```python
from build123d import *
from build123d.topology import SkipClean

# Parameters (mm, degrees)
SKETCH_1_R           = 15
SKETCH_1_R_2         = 4
SKETCH_1_R_3         = 1.6
EXTRUDE_1_DEPTH      = 4
EXTRUDE_START        = -4
EXTRUDE_3_DEPTH      = 4
EXTRUDE_4_DEPTH      = 8
EXTRUDE_4_DEPTH_BACK = 12
CUT_EXTRUDE_1_DEPTH  = 46


with BuildPart() as part:
    # 草图1 → 凸台-拉伸1 (new body)
    with BuildSketch(Plane.XY):
        Circle(SKETCH_1_R)
        Circle(SKETCH_1_R_2, mode=Mode.SUBTRACT)
        with Locations((0, 8)):
            Circle(SKETCH_1_R_3, mode=Mode.SUBTRACT)
        with Locations((6.92820323, 4)):
            Circle(SKETCH_1_R_3, mode=Mode.SUBTRACT)
        with Locations((6.92820323, -4)):
            Circle(SKETCH_1_R_3, mode=Mode.SUBTRACT)
        with Locations((0, -8)):
            Circle(SKETCH_1_R_3, mode=Mode.SUBTRACT)
        with Locations((-6.92820323, -4)):
            Circle(SKETCH_1_R_3, mode=Mode.SUBTRACT)
        with Locations((-6.92820323, 4)):
            Circle(SKETCH_1_R_3, mode=Mode.SUBTRACT)
    extrude(amount=EXTRUDE_1_DEPTH)

    # 草图2 → 凸台-拉伸3 (add)
    with BuildSketch(Plane.XY.offset(4).offset(EXTRUDE_START)):
        with BuildLine():
            Line((16.8, 85), (16.8, 54.159799849))
            ThreePointArc((16.8, 54.159799849), (15.83854762, 48.033324147), (13.046629547, 42.49587991))
            ThreePointArc((13.046629547, 42.49587991), (7.420814059, 25.504374344), (12.472191289, 8.333333333))
            ThreePointArc((12.472191289, 8.333333333), (-5.937882388, 13.774670695), (-14.621995932, -3.346226976))
            ThreePointArc((-14.621995932, -3.346226976), (-15.737901413, 44.738127218), (2.117573463, 89.398315084))
            ThreePointArc((2.117573463, 89.398315084), (11.095712057, 92.663530919), (16.8, 85))
        make_face()
    extrude(amount=EXTRUDE_3_DEPTH)

    # 草图3 → 凸台-拉伸4 (add, two sides: drawn at the far end of the back side and taken through both)
    with SkipClean():  # the faces are left unmerged after this step: merging them gives an invalid solid
        with BuildSketch(Plane.XY.offset(4).offset(-EXTRUDE_4_DEPTH_BACK)):
            with BuildLine():
                Line((16.8, 54.159799849), (16.8, 85))
                ThreePointArc((16.8, 85), (11.095712057, 92.663530919), (2.117573463, 89.398315084))
                ThreePointArc((2.117573463, 89.398315084), (-11.916705707, 60.059804871), (-17.55757213, 28.030290369))
                ThreePointArc((-17.55757213, 28.030290369), (-15.746673, 24.526996644), (-11.810776072, 24.27973576))
                ThreePointArc((-11.810776072, 24.27973576), (-4.386649325, 26.64127076), (3.402697603, 26.784727906))
                ThreePointArc((3.402697603, 26.784727906), (6.286614818, 27.53779516), (7.849127177, 30.076031539))
                ThreePointArc((7.849127177, 30.076031539), (9.742150736, 36.581291134), (13.046629547, 42.49587991))
                ThreePointArc((13.046629547, 42.49587991), (15.83854762, 48.033324147), (16.8, 54.159799849))
            make_face()
        extrude(amount=EXTRUDE_4_DEPTH + EXTRUDE_4_DEPTH_BACK)
    add(part.part.scale(1), mode=Mode.REPLACE)  # the faces are merged on a copy

    # 草图5 → 切除-拉伸1 (cut)
    with BuildSketch(Plane(origin=(0, 0, -8), x_dir=(-1, 0, 0), z_dir=(0, 0, -1))):
        with BuildLine():
            Line((-12.8, 69.762395693), (-12.8, 60.082793322))
            ThreePointArc((-12.8, 60.082793322), (-11.947152873, 58.444489233), (-10.115959713, 58.20340808))
            Line((-10.115959713, 58.20340808), (0.167044148, 61.946115404))
            ThreePointArc((0.167044148, 61.946115404), (1.475393257, 63.65118916), (0.483003861, 65.557551453))
            Line((0.483003861, 65.557551453), (-9.8, 71.494446501))
            ThreePointArc((-9.8, 71.494446501), (-11.8, 71.494446501), (-12.8, 69.762395693))
        make_face()
        with BuildLine():
            Line((-11.8, 78.422649731), (-1.206357847, 72.306407582))
            ThreePointArc((-1.206357847, 72.306407582), (1.162211364, 72.580028303), (1.585705551, 74.926438557))
            ThreePointArc((1.585705551, 74.926438557), (-1.749223409, 81.170317372), (-5.458786731, 87.199157542))
            ThreePointArc((-5.458786731, 87.199157542), (-9.947856029, 88.83176546), (-12.8, 85))
            Line((-12.8, 85), (-12.8, 80.154700538))
            ThreePointArc((-12.8, 80.154700538), (-12.532050808, 79.154700538), (-11.8, 78.422649731))
        make_face()
        with BuildLine():
            Line((5.01005666, 58.38793894), (-5.776995128, 54.461773174))
            ThreePointArc((-5.776995128, 54.461773174), (-7.091051284, 52.669626708), (-5.938191364, 50.769772359))
            Line((-5.938191364, 50.769772359), (7.453099332, 44.525310955))
            ThreePointArc((7.453099332, 44.525310955), (9.539258698, 44.76945259), (10.256783773, 46.743490028))
            ThreePointArc((10.256783773, 46.743490028), (9.051891671, 51.949605837), (7.60645214, 57.094128298))
            ThreePointArc((7.60645214, 57.094128298), (6.586103601, 58.298616303), (5.01005666, 58.38793894))
        make_face()
        with BuildLine():
            Line((-2.123332063, 32.377143259), (7.681973135, 35.004466868))
            ThreePointArc((7.681973135, 35.004466868), (9.156724441, 36.762007035), (8.009571568, 38.748934095))
            Line((8.009571568, 38.748934095), (-5.543860738, 45.069003373))
            ThreePointArc((-5.543860738, 45.069003373), (-7.869208523, 44.601479118), (-8.112845962, 42.242144033))
            ThreePointArc((-8.112845962, 42.242144033), (-6.056960525, 38.136767143), (-4.572948137, 33.791828527))
            ThreePointArc((-4.572948137, 33.791828527), (-3.641181599, 32.577066199), (-2.123332063, 32.377143259))
        make_face()
    extrude(amount=-CUT_EXTRUDE_1_DEPTH, mode=Mode.SUBTRACT)


solid = part.part
```
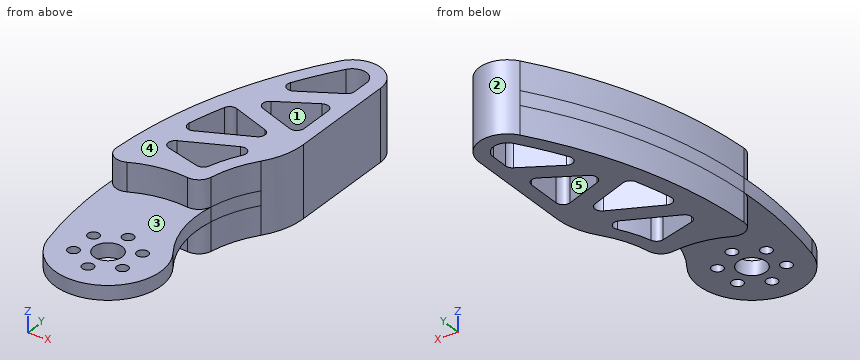
For this review, take the finished solid that the model builds, in its own axes (mm). Face numbers are marked on the shaded views. A direction names the side the tool comes from. Round coordinates to 2 decimals unless told otherwise and drop trailing zeros. Write each loop counter-clockwise with the first axis right and the second up, starting at its lowest first coordinate (ties: lowest second). Pieces come first, ordered by that corner, then holes. Notation, with made-up numbers: (77, 6) -> (130, 6) arc R34 ccw to (130, 36) -> close; hole circle Ø3 at (46, 46). An arc over 180 degrees is marked (long way). Use one line per item in the form item = value.
Q1. Consider section C-C (x = -3). State the section outline as (y, z) points.
Resolved:
outline = (-14.7, 0) -> (-2.65, 0) -> (-2.65, 4) -> (-14.7, 4) -> close; (2.65, 0) -> (26.83, 0) -> (26.83, -8) -> (33.75, -8) -> (33.75, 12) -> (26.83, 12) -> (26.83, 4) -> (2.65, 4) -> close; (41.08, -8) -> (46.6, -8) -> (46.6, 12) -> (41.08, 12) -> close; (57.66, -8) -> (80.87, -8) -> (80.87, 12) -> (57.66, 12) -> close
Q2. Clearance check with flat-ended pins moving along their axes: pin 1 Ø3 at (x, y) = (6.93, -4) entering from -Z; pin 2 Ø3.5 at (x, y) = (6.93, 4) entering from +Z; pin 3 Ø16.5 at (x, y) = (-4.5, 10) entering from -Z; pin 4 Ø6 at (y, z) = (6, -2) entering from +X. State where each tip first meets the part, or that it passes through.
Resolved:
pin_1 = through
pin_2 = 4
pin_3 = 0
pin_4 = 14.52
Q3. Machinability: for the marked faces 4 and 5, which of the approach directions +Z, -Z, +X, -X, +Y, -Y give a long, thin tool a straight path to every point of the face, cutting with its end or side? Answer none if there is none.
Resolved:
face_4 = +Z, +X, -X, +Y, -Y
face_5 = +Z, -Z
Q4. Consider section A-A (y = 0). State the section outline as (x, z) points, then the cut area to 3 significant figures.
Resolved:
outline = (-15.34, 0) -> (-4, 0) -> (-4, 4) -> (-15.34, 4) -> close; (4, 0) -> (15, 0) -> (15, 4) -> (4, 4) -> close
area = 89.4 mm²
Q5. To check wall thickness, follow probe 1 along Y at (x, z) = (10.5, 7.25); probe 2 along Y at (x, z) = (-3.5, -2); probe 3 along X at (y, z) = (79.5, 2). State the ranges of each line that lie inside material, in increasing order. Write a range as from..to.
Resolved:
probe_1 = 38.25..58.11, 71.74..77.67, 88.62..92.82
probe_2 = 26.77..33.88, 40.85..46.37, 57.84..79.95
probe_3 = -3.74..0.81, 12.69..16.8
Q6. Consider section B-B (z = -4). State how many separate pieces and enclosed holes the cut face has, then the cut area to 3 significant figures.
Resolved:
separate_pieces = 1
enclosed_holes = 4
area = 1,110 mm²
Q7. The part is to be moulded in two halves that separate along Y. For the marked faces 1, 2 and 3, say which applies: released by +Y, released by -Y, zero draft, split by the parting line, or undercut.
Resolved:
face_1 = undercut
face_2 = released by +Y
face_3 = zero draft
